Design review of the part built by this model. Coordinates are the model's own, in mm. A direction names the side the tool comes from. Coordinates: 2 decimals unless noted, no trailing zeros. Write each loop counter-clockwise with the first axis right and the second up, starting at its lowest first coordinate (ties: lowest second). Pieces come first, ordered by that corner, then holes. Notation, with made-up numbers: M 21.25,60.25 L 25.25,60.25 A6 cw 25.25,69.25 Z; hole C 61.5,-11 d7. An arc over 180 degrees is marked long. One line per question, with ' | ' between items.
from build123d import *

# Parameters (mm, degrees)
BOSS_EXTRUDE1_DEPTH = 20
FILLET1_R           = 3
SKETCH3_R           = 2
CUT_EXTRUDE1_DEPTH  = 52.909473261
SKETCH4_R           = 2
CUT_EXTRUDE2_DEPTH  = 51.587344223


with BuildPart() as part:
    # Sketch1 → Boss-Extrude1 (new body)
    with BuildSketch(Plane(origin=(0, 0, 0), x_dir=(1, 0, 0), z_dir=(0, 1, 0))):
        Polygon((-13.644859813, 18.355140187), (-13.644859813, -21.644859813), (26.355140187, -21.644859813), (26.355140187, -23.644859813), (-15.644859813, -23.644859813), (-15.644859813, 18.355140187), align=None)
    extrude(amount=BOSS_EXTRUDE1_DEPTH)

    # Fillet1
    fillet1_edges = [part.edges().sort_by_distance(p)[0] for p in [
        (-13.644859813, 10, 21.644859813),
        (-15.644859813, 10, 23.644859813),
        (26.355140187, 20, 22.644859813),
        (-14.644859813, 20, -18.355140187),
        (26.355140187, 0, 22.644859813),
        (-14.644859813, 0, -18.355140187),
    ]]
    fillet(fillet1_edges, radius=FILLET1_R)

    # Sketch3 → Cut-Extrude1 (cut, through all)
    with BuildSketch(Plane(origin=(0, 0, 21.644859813), x_dir=(-1, 0, 0), z_dir=(0, 0, -1))):
        with Locations((-1.355140187, 10)):
            Circle(SKETCH3_R)
        with Locations((-16.355140187, 10)):
            Circle(SKETCH3_R)
    extrude(amount=-CUT_EXTRUDE1_DEPTH, mode=Mode.SUBTRACT)

    # Sketch4 → Cut-Extrude2 (cut, through all)
    with BuildSketch(Plane(origin=(-13.644859813, 0, 0), x_dir=(0, 0, -1), z_dir=(1, 0, 0))):
        with Locations((8.355140187, 10)):
            Circle(SKETCH4_R)
        with Locations((-6.644859813, 10)):
            Circle(SKETCH4_R)
    extrude(amount=-CUT_EXTRUDE2_DEPTH, mode=Mode.SUBTRACT)


solid = part.part
1. Take a section at B-B (z = -9). Write out the cut boundary in (x, y), then the cut area to 3 significant figures.
Answer sheet:
outline: M -15.64,0 L -13.64,0 L -13.64,8.11 L -15.64,8.11 Z; M -15.64,11.89 L -13.64,11.89 L -13.64,20 L -15.64,20 Z | area: 32.4 mm^2
2. Take a section at A-A (y = 10). Write out the cut boundary in (x, z), then the cut area to 3 significant figures.
Answer sheet:
outline: M -15.64,-18.36 L -13.64,-18.36 L -13.64,-10.36 L -15.64,-10.36 Z; M -15.64,-6.36 L -13.64,-6.36 L -13.64,4.64 L -15.64,4.64 Z; M -15.64,8.64 L -13.64,8.64 L -13.64,18.64 A3 cw -10.64,21.64 L -0.64,21.64 L -0.64,23.64 L -12.64,23.64 A3 ccw -15.64,20.64 Z; M 3.36,21.64 L 14.36,21.64 L 14.36,23.64 L 3.36,23.64 Z; M 18.36,21.64 L 26.36,21.64 L 26.36,23.64 L 18.36,23.64 Z | area: 132 mm^2
3. To check wall thickness, follow line 1 along X through (y, z) = (1.5, 17); line 2 along Z through (x, y) = (17, 7.5); line 3 along X through (y, z) = (14.75, 19.5). State the ranges of each line that lie inside material, in increasing order. Write a range as [from, to].
Answer sheet:
line 1: [-15.64, -13.64] | line 2: [21.64, 23.64] | line 3: [-15.64, -13.52]
4. Draft analysis for pull direction X (two halves, no side actions). For faces 3 (the face through (-15.645, 10, 1)), 4 (the face through (-6, 0, 23)), 5 (the face through (1.616, 11.983, 22.631)), state which applies: pulls with the +X half, pulls with the -X half, needs draft (parallel to the pull), parting line crosses it, or undercut.
Answer sheet:
face 3: pulls with the -X half | face 4: needs draft | face 5: undercut
5. Take a section at D-D (x = 22). Write out the cut boundary in (y, z), then the cut area to 3 significant figures.
Answer sheet:
outline: M 0,21.64 L 20,21.64 L 20,23.64 L 0,23.64 Z | area: 40.0 mm^2
6. Take a section at C-C (y = 15.25). Write out the cut boundary in (x, z).
Answer sheet:
outline: M -15.64,-18.36 L -13.64,-18.36 L -13.64,18.64 A3 cw -10.64,21.64 L 26.36,21.64 L 26.36,23.64 L -12.64,23.64 A3 ccw -15.64,20.64 Z
7. Insertion check: pin 1 Ø1.5 at (y, z) = (9, -5) entering from +X; pin 2 Ø4.5 at (x, y) = (1.36, 10) entering from -Z; pin 3 Ø6 at (y, z) = (15.5, 16.5) entering from +X. Each pin has a flat end and moves straight along its axis. Give the tip position at first contact, or say it passes through.
Answer sheet:
pin 1: x = -13.64 | pin 2: z = 21.64 | pin 3: x = -13.52
8. Tool access review of faces 1 (the face through (8, 10, 21.645)), 2 (the face through (-14.6, 0.9, -17.5)): name each direction out of +Z, -Z, +X, -X, +Y, -Y from which nothing blocks a thin tool from reaching the whole face with its end or side.
Answer sheet:
face 1: -Z, +X, +Y, -Y | face 2: -Z, +X, -X, -Y
